Could you check a few things on this model? Use its own coordinates, in mm. A direction names the side the tool comes from. Coordinates: 2 decimals unless noted, no trailing zeros. Write each loop counter-clockwise with the first axis right and the second up, starting at its lowest first coordinate (ties: lowest second). Pieces come first, ordered by that corner, then holes. Notation, with made-up numbers: M 76,-7.5 L 95,-7.5 A17 cw 95,17.5 Z; hole C 85,-4.5 d11. An arc over 180 degrees is marked long. Answer as CSV lines item,"result". Start each with the question number.
Item 1: We'd pull the mould along Z, two halves only. Please class faces 4 (the flat face through (15, 0, 2)), 5 (the flat face through (0, 0, -1)), 6 (the flat face through (-13, -13, 1)): +Z half, -Z half, draft (parallel to the pull), parting line (faces both ways), or undercut.
Item 2: If I drill on line 1 along Z through (x, y) = (-1, 5.25); line 2 along X through (y, z) = (-0.25, 0.9), over which ranges is the centre line in solid material (lowest first)? Write a range as [from, to].
Item 3: I'm going to push flat-ended pins straight in: P1, Ø0.7, axis at y = 2.5, z = 0.5, coming from the -X side; P2, Ø0.8, axis at x = -13, z = 0.5, coming from the +Y side; P3, Ø0.8, axis at x = 7.5, z = 1, coming from the -Y side. Where does each tip first touch, or does it pass through?
Item 4: Suppose I cut it at D-D, the plane y = -5. Write out the boundary of the cut face in (x, z).
Item 5: Suppose I cut it at A-A, the plane x = 1. Write out the boundary of the cut face in (y, z).
Item 6: Suppose I cut it at C-C, the plane x = -8. Write out the boundary of the cut face in (y, z).
Item 7: On a 3-axis mill with a long thin cutter (end or side, diameter ignored), from which of +Z, -Z, +X, -X, +Y, -Y can I reach the whole of each face in a straight line? I mean faces 1 (the flat face through (11.5, 10, 1)), 2 (the flat face through (-8, 12, 1)), 3 (the flat face through (-13.5, 10, 1)). Say none if no direction works.
```python
from build123d import *

# Parameters (mm, degrees)
F0_W     = 30
F0_H     = 30
F1_DEPTH = 1
F2_W     = 1.5
F2_H     = 1.4999990595
F3_DEPTH = 1.5
F4_W     = 30
F4_H     = 30
F5_DEPTH = 1


with BuildPart() as f1:
    # F0 (on Top) → F1 (new body)
    with BuildSketch(Plane.XY):
        Rectangle(F0_W, F0_H)
    extrude(amount=-F1_DEPTH)

    # F2 (on face) → F3 (join)
    with BuildSketch(Plane.XY):
        with Locations((-12.75, 12.7500004702)):
            Rectangle(F2_W, F2_H)
        with Locations((-10.25, 12.7500004702)):
            Rectangle(F2_W, F2_H)
        with Locations((-7.75, 12.7500004702)):
            Rectangle(F2_W, F2_H)
        with Locations((-5.25, 12.7500004702)):
            Rectangle(F2_W, F2_H)
        with Locations((-2.75, 12.7500004702)):
            Rectangle(F2_W, F2_H)
        with Locations((-0.25, 12.7500004702)):
            Rectangle(F2_W, F2_H)
        with Locations((2.25, 12.7500004702)):
            Rectangle(F2_W, F2_H)
        with Locations((4.75, 12.7500004702)):
            Rectangle(F2_W, F2_H)
        with Locations((7.25, 12.7500004702)):
            Rectangle(F2_W, F2_H)
        with Locations((9.75, 12.7500004702)):
            Rectangle(F2_W, F2_H)
        with Locations((12.25, 12.7500004702)):
            Rectangle(F2_W, F2_H)
        with Locations((12.25, 10.2500004702)):
            Rectangle(F2_W, F2_H)
        with Locations((-12.75, 10.2500004702)):
            Rectangle(F2_W, F2_H)
        with Locations((12.25, 7.7500004702)):
            Rectangle(F2_W, F2_H)
        with Locations((-12.75, 7.7500004702)):
            Rectangle(F2_W, F2_H)
        with Locations((12.25, 5.2500004702)):
            Rectangle(F2_W, F2_H)
        with Locations((-12.75, 5.2500004702)):
            Rectangle(F2_W, F2_H)
        with Locations((12.25, 2.7500004702)):
            Rectangle(F2_W, F2_H)
        with Locations((-12.75, 2.7500004702)):
            Rectangle(F2_W, F2_H)
        with Locations((12.25, 0.2500004702)):
            Rectangle(F2_W, F2_H)
        with Locations((-12.75, 0.2500004702)):
            Rectangle(F2_W, F2_H)
        with Locations((12.25, -2.2499995298)):
            Rectangle(F2_W, F2_H)
        with Locations((-12.75, -2.2499995298)):
            Rectangle(F2_W, F2_H)
        with Locations((12.25, -4.7499995298)):
            Rectangle(F2_W, F2_H)
        with Locations((-12.75, -4.7499995298)):
            Rectangle(F2_W, F2_H)
        with Locations((12.25, -7.2499995298)):
            Rectangle(F2_W, F2_H)
        with Locations((-12.75, -7.2499995298)):
            Rectangle(F2_W, F2_H)
        with Locations((12.25, -9.7499995298)):
            Rectangle(F2_W, F2_H)
        with Locations((-12.75, -9.7499995298)):
            Rectangle(F2_W, F2_H)
        with Locations((-0.25, -12.2499995298)):
            Rectangle(F2_W, F2_H)
        with Locations((9.75, -12.2499995298)):
            Rectangle(F2_W, F2_H)
        with Locations((-5.25, -12.2499995298)):
            Rectangle(F2_W, F2_H)
        with Locations((-10.25, -12.2499995298)):
            Rectangle(F2_W, F2_H)
        with Locations((4.75, -12.2499995298)):
            Rectangle(F2_W, F2_H)
        with Locations((-2.75, -12.2499995298)):
            Rectangle(F2_W, F2_H)
        with Locations((7.25, -12.2499995298)):
            Rectangle(F2_W, F2_H)
        with Locations((2.25, -12.2499995298)):
            Rectangle(F2_W, F2_H)
        with Locations((12.25, -12.2499995298)):
            Rectangle(F2_W, F2_H)
        with Locations((-7.75, -12.2499995298)):
            Rectangle(F2_W, F2_H)
        with Locations((-12.75, -12.2499995298)):
            Rectangle(F2_W, F2_H)
    extrude(amount=F3_DEPTH)

    # F4 (on face) → F5 (join)
    with BuildSketch(Plane.XY.offset(1.5)):
        Rectangle(F4_W, F4_H)
    extrude(amount=F5_DEPTH)


solid = f1.part
```
Ans:
1,face 4,"draft"
1,face 5,"-Z half"
1,face 6,"undercut"
2,line 1,"z = [-1, 0], [1.5, 2.5]"
2,line 2,"x = [-13.5, -12], [11.5, 13]"
3,P1,"stops at x = -13.5"
3,P2,"stops at y = 13.5"
3,P3,"stops at y = -13"
4,outline,"M -15,-1 L 15,-1 L 15,0 L 13,0 L 13,1.5 L 15,1.5 L 15,2.5 L -15,2.5 L -15,1.5 L -13.5,1.5 L -13.5,0 L -15,0 Z; hole M -12,0 L 11.5,0 L 11.5,1.5 L -12,1.5 Z"
5,outline,"M -15,-1 L 15,-1 L 15,0 L -15,0 Z; M -15,1.5 L 15,1.5 L 15,2.5 L -15,2.5 Z"
6,outline,"M -15,-1 L 15,-1 L 15,0 L 13.5,0 L 13.5,1.5 L 15,1.5 L 15,2.5 L -15,2.5 L -15,1.5 L -13,1.5 L -13,0 L -15,0 Z; hole M -11.5,0 L 12,0 L 12,1.5 L -11.5,1.5 Z"
7,face 1,"+Y, -Y"
7,face 2,"+X, -X"
7,face 3,"-X, +Y, -Y"
